The model under review builds one solid part; all positions refer to its coordinate system, in mm. Face numbers are marked on the shaded views. A direction names the side the tool comes from. Round coordinates to 2 decimals unless told otherwise and drop trailing zeros. Loops run counter-clockwise (first coordinate to the right, second up) from the corner with the lowest first, then second, coordinate; pieces in that order, holes last. Notation, with made-up numbers: (51.25, 10.25) -> (60.25, 10.25) arc R23 ccw to (60.25, 19.25) -> close; hole circle Ø3 at (-3.5, 26). An arc over 180 degrees is marked (long way). Write each question's results on one line, items separated by ' | '. Start each with the question number.
Item 1: For L1, parallel to Y at x = 2, z = 8; L2, parallel to Y at x = -5, z = 62.5; L3, parallel to Z at x = 16.5, y = -20, list the stretches that pass through material, from the lowest coordinate up. Write a range as from..to.
Item 2: Tool access review of the marked faces 1, 2, 3 and 4: name each direction out of +Z, -Z, +X, -X, +Y, -Y from which nothing blocks a thin tool from reaching the whole face with its end or side.
Item 3: We need section D-D (y = 5). Give the boundary of the cut face in (x, z).
Item 4: We need section A-A (x = 15). Give the boundary of the cut face in (y, z).
Item 5: Clearance check with flat-ended pins moving along their axes: pin 1 Ø10 at (y, z) = (3, 41.5) entering from +X; pin 2 Ø5 at (x, z) = (11.5, 69) entering from -Y; pin 3 Ø13 at (y, z) = (-7, 80.5) entering from +X; pin 4 Ø8 at (x, y) = (-11.5, -19) entering from -Z. State where each tip first meets the part, or that it passes through.
Item 6: Mouldability with a two-part tool opening along Y and no side actions: class the marked faces 5, 6 and 7 as pulls with the +Y half, pulls with the -Y half, needs draft (parallel to the pull), parting line crosses it, or undercut.
Item 7: We need section C-C (z = 39.5). Give the boundary of the cut face in (x, y).
Item 8: We need section B-B (y = 25). Give the boundary of the cut face in (x, z), and give its area (3 significant figures).
from build123d import *

# Parameters (mm, degrees)
F0_W     = 50.8
F0_H     = 86.36
F1_DEPTH = 25.4
F2_W     = 38.1
F2_H     = 76.2
F3_DEPTH = 101.6
F4_W     = 50.8
F4_H     = 86.36
F4_W_2   = 38.1
F4_H_2   = 76.2
F5_DEPTH = 12.7
F6_W     = 12.7
F6_H     = 21.59
F7_DEPTH = 76.2


with BuildPart() as f1:
    # F0 (on Top) → F1 (new body)
    with BuildSketch(Plane.XY):
        Rectangle(F0_W, F0_H)
    extrude(amount=F1_DEPTH)

    # F2 (on face) → F3 (cut)
    with BuildSketch(Plane.XY.offset(25.4)):
        Rectangle(F2_W, F2_H)
    extrude(amount=-F3_DEPTH, mode=Mode.SUBTRACT)

    # F4 (on face) → F5 (join)
    with BuildSketch(Plane.XY.offset(25.4)):
        Rectangle(F4_W, F4_H)
        Rectangle(F4_W_2, F4_H_2, mode=Mode.SUBTRACT)
        Rectangle(F4_W_2, F4_H_2)
    extrude(amount=F5_DEPTH)

    # F6 (on face) → F7 (join)
    with BuildSketch(Plane.XY.offset(38.1)):
        with Locations((-19.05, 10.795)):
            Rectangle(F6_W, F6_H)
        with Locations((-6.35, 10.795)):
            Rectangle(F6_W, F6_H)
        with Locations((-19.05, -10.795)):
            Rectangle(F6_W, F6_H)
        Polygon((12.7, 21.59), (0, 21.59), (0, 0), (0, -21.59), (12.7, -21.59), (12.7, 0), align=None)
        with Locations((-6.35, -10.795)):
            Rectangle(F6_W, F6_H)
    extrude(amount=F7_DEPTH)


solid = f1.part
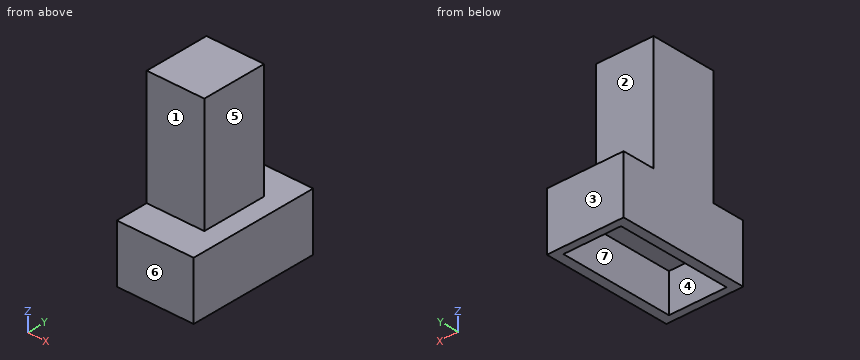
Here are the results:
1) L1: y = -43.18..-38.1, 38.1..43.18 | L2: y = -21.59..21.59 | L3: z = 25.4..38.1
2) face 1: +Z, +X, -X, -Y | face 2: +Z, +X, -X, +Y | face 3: +Z, -Z, +X, -X, +Y | face 4: -Z
3) outline: (-25.4, 0) -> (-19.05, 0) -> (-19.05, 25.4) -> (19.05, 25.4) -> (19.05, 0) -> (25.4, 0) -> (25.4, 38.1) -> (12.7, 38.1) -> (12.7, 114.3) -> (-25.4, 114.3) -> close
4) outline: (-43.18, 0) -> (-38.1, 0) -> (-38.1, 25.4) -> (38.1, 25.4) -> (38.1, 0) -> (43.18, 0) -> (43.18, 38.1) -> (-43.18, 38.1) -> close
5) pin 1: stops at x = 25.4 | pin 2: stops at y = -21.59 | pin 3: stops at x = 12.7 | pin 4: stops at z = 25.4
6) face 5: needs draft | face 6: pulls with the -Y half | face 7: undercut
7) outline: (-25.4, -21.59) -> (12.7, -21.59) -> (12.7, 21.59) -> (-25.4, 21.59) -> close
8) outline: (-25.4, 0) -> (-19.05, 0) -> (-19.05, 25.4) -> (19.05, 25.4) -> (19.05, 0) -> (25.4, 0) -> (25.4, 38.1) -> (-25.4, 38.1) -> close | area: 968 mm2
